Geometry: final body of the model. Coordinates: model frame, mm. Coordinates: 2 decimals unless noted, no trailing zeros. Write each loop counter-clockwise with the first axis right and the second up, starting at its lowest first coordinate (ties: lowest second). Pieces come first, ordered by that corner, then holes. Notation, with made-up numbers: (13.5, 43) - (62.5, 43) arc R24 cw to (62.5, 66) - close; hole circle Ø2 at (40, 84.25). An arc over 180 degrees is marked (long way). Put each result on its own line as item: value.
```python
from build123d import *

# Parameters (mm, degrees)
BOSS_EXTRUDE1_DEPTH = 700
SHELL1_T            = -4


with BuildPart() as part:
    # Sketch2 → Boss-Extrude1 (new body)
    with BuildSketch(Plane(origin=(0, 0, 0), x_dir=(0, 0, -1), z_dir=(1, 0, 0))):
        Polygon((0, 0), (0, 65.147186258), (84.852813742, 150), (884.852813742, 150), (884.852813742, 0), align=None)
    extrude(amount=BOSS_EXTRUDE1_DEPTH)

    # Shell1
    shell1_openings = [part.faces().sort_by_distance(p)[0] for p in [
        (350, 150, -484.852813742),
    ]]
    offset(amount=SHELL1_T, openings=shell1_openings, kind=Kind.INTERSECTION)


solid = part.part
```
1. Pin query (flat end, axial travel): pin 1 Ø3 at (x, z) = (270, -98.5) entering from +Y. Return the tip coordinate at first contact, or that it passes through.
Answer below:
pin 1: stops at y = 4
2. Section query B-B (z = -507.5). Return loops of the section in (x, y).
Answer below:
outline: (0, 0) - (700, 0) - (700, 150) - (696, 150) - (696, 4) - (4, 4) - (4, 150) - (0, 150) - close
3. Section query C-C (x = 252.5). Return loops of the section in (y, z).
Answer below:
outline: (0, -884.85) - (150, -884.85) - (150, -880.85) - (4, -880.85) - (4, -4) - (63.49, -4) - (150, -90.51) - (150, -84.85) - (65.15, 0) - (0, 0) - close
4. Section query A-A (y = 29.5). Return loops of the section in (x, z).
Answer below:
outline: (0, -884.85) - (700, -884.85) - (700, 0) - (0, 0) - close; hole (4, -880.85) - (696, -880.85) - (696, -4) - (4, -4) - close
5. Ray query, probe 1 along X at (y, z) = (54.5, -588); probe 2 along Z at (x, y) = (564.5, 30.5); probe 3 along Y at (x, z) = (349, -709.5). Return the intervals inside material, ascending. Write a range as from..to.
Answer below:
probe 1: x = 0..4, 696..700
probe 2: z = -884.85..-880.85, -4..0
probe 3: y = 0..4
6. Section query D-D (z = -59.5). Return loops of the section in (x, y), then the cut area to 3 significant figures.
Answer below:
outline: (0, 0) - (700, 0) - (700, 124.65) - (0, 124.65) - close; hole (4, 4) - (696, 4) - (696, 118.99) - (4, 118.99) - close
area: 7,680 mm²
7. Mould query, pull axis Y, two halves, no side actions, for faces 1 (the flat face through (345, 33, -4)), 2 (the flat face through (345, 78, -880.853)), 3 (the flat face through (345.1, 106.98, -41.83)), 4 (the flat face through (345.16, 106.14, -46.65)). Classes: +Y half, -Y half, draft (parallel to the pull), parting line (faces both ways), or undercut.
Answer below:
face 1: undercut
face 2: draft
face 3: +Y half
face 4: undercut
